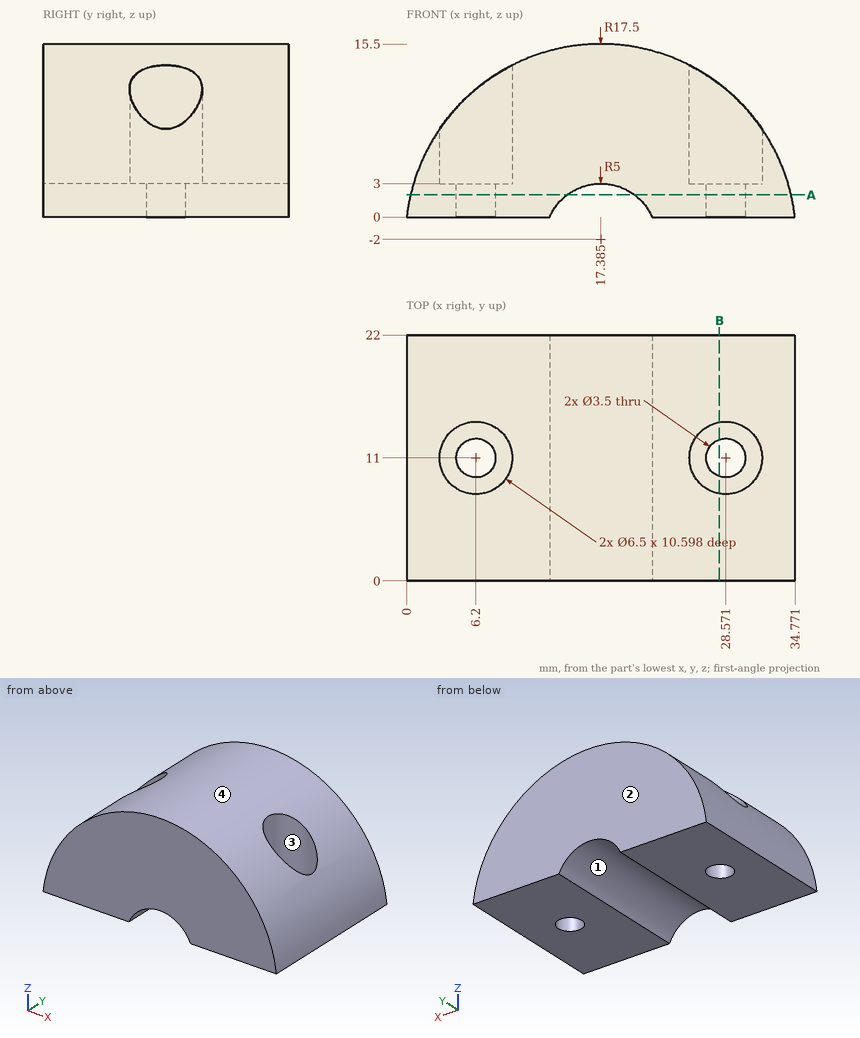
Here's the drawing with two shaded views (mm, measured from the low corner). I have some questions. Round coordinates to 2 decimals unless told otherwise and drop trailing zeros. Loops run counter-clockwise (first coordinate to the right, second up) from the corner with the lowest first, then second, coordinate; pieces in that order, holes last. Notation, with made-up numbers: (-37, 1.25) -> (7, 1.25) arc R9 cw to (7, 11.25) -> close; hole circle Ø11 at (-13.5, -1). An arc over 180 degrees is marked (long way). Answer as CSV lines item,"result". Start each with the question number.
1. I need wall thicknesses on probe 1 along X at (y, z) = (8.25, 3.5) (1 decimal); probe 2 along X at (y, z) = (10, 6.5); probe 3 along Y at (x, z) = (27, 12.25) (1 decimal). Which ranges of each line are inside material? Lowest first, please. Write a range as from..to.
2. I'm going to push flat-ended pins straight in: P1, Ø5, axis at x = 9, y = 16, coming from the +Z side; P2, Ø1.5, axis at y = 4.5, z = 14, coming from the -X side; P3, Ø6, axis at y = 19, z = 10, coming from the -X side. Where does each tip first touch, or does it pass through?
3. Imagine slicing it at B-B on x = 28. Write out the boundary of the cut face in (y, z) (1 decimal), plus the area to 3 significant figures.
4. If we mould it in two halves opening along X, with no side actions, what happens to the marked faces 1, 2, 3 and 4? For each: pulls with the +X half, pulls with the -X half, needs draft (parallel to the pull), parting line crosses it, or undercut.
5. Imagine slicing it at A-A on z = 2. State how many separate pieces and enclosed holes the cut face has.
Solution:
1,probe 1,"0.8..4.5, 7.9..26.8, 30.3..34"
1,probe 2,"2.09..3.11, 9.29..25.48, 31.66..32.68"
1,probe 3,"0..8.2, 13.8..22"
2,P1,"z = 14.48"
2,P2,"x = 8.8"
2,P3,"x = 2.38"
3,outline,"(0, 0) -> (9.3, 0) -> (9.3, 3) -> (7.8, 3) -> (7.8, 11.9) -> (0, 11.9) -> close; (12.7, 0) -> (22, 0) -> (22, 11.9) -> (14.2, 11.9) -> (14.2, 3) -> (12.7, 3) -> close"
3,area,"195 mm²"
4,face 1,"undercut"
4,face 2,"needs draft"
4,face 3,"undercut"
4,face 4,"parting line crosses it"
5,separate pieces,"2"
5,enclosed holes,"2"
